Here's how the part is built. I have some questions about the finished solid (model axes, mm). A direction names the side the tool comes from. Give positions to 0.01 mm unless a question says otherwise; leave off trailing zeros. Write each loop counter-clockwise with the first axis right and the second up, starting at its lowest first coordinate (ties: lowest second). Pieces come first, ordered by that corner, then holes. Notation, with made-up numbers: (45, 22.25) -> (88, 22.25) arc R21 cw to (88, 34.25) -> close; hole circle Ø11 at (5, -2). An arc over 180 degrees is marked (long way). Use one line per item in the form item = value.
```python
from build123d import *

# Parameters (mm, degrees)
F0_W      = 11.8
F0_H      = 21.82
F3_W      = 1.2
F3_H      = 40
F4_DEPTH  = 26
F5_R      = 11.8
F6_DEPTH  = 30
F2_W      = 11.2
F2_H      = 8
F9_W      = 21
F9_H      = 12
F10_DEPTH = 20
F11_R     = 5.99999
F13_R     = 1.2
F14_R     = 3
F15_DEPTH = 12.5


# Not quite as in the source:
# - a fillet or chamfer is up to 0.001 mm smaller than in the source, because OpenCascade refuses the exact size


with BuildPart() as f1:
    # F0 (on Front) → F1 (revolve)
    with BuildSketch(Plane.XZ):
        with Locations((5.9, 10.91)):
            Rectangle(F0_W, F0_H)
    revolve(axis=Axis((0, 0, 10.91), (0, 0, 1)))


with BuildPart() as f4:
    # F3 (on Top) → F4 (new body)
    with BuildSketch(Plane.XY):
        with Locations((5.2, 0)):
            Rectangle(F3_W, F3_H)
    extrude(amount=F4_DEPTH)


with BuildPart() as f6_tool:
    # F5 (on Top) → F6 (new body)
    with BuildSketch(Plane.XY):
        Circle(F5_R)
    extrude(amount=F6_DEPTH)


with BuildPart() as f1_1:
    add(f1.part)

    # F6: intersect by f6_tool
    add(f6_tool.part, mode=Mode.INTERSECT)


with BuildPart() as f4_1:
    add(f4.part)

    # F6: intersect by f6_tool
    add(f6_tool.part, mode=Mode.INTERSECT)

    # F7: union F1
    add(f1_1.part)

    # F2 (on Front) → F8 (revolve, cut)
    with BuildSketch(Plane.XZ):
        with Locations((5.6, 4)):
            Rectangle(F2_W, F2_H)
    revolve(axis=Axis((0, 0, 4), (0, 0, 1)), mode=Mode.SUBTRACT)


with BuildPart() as f10:
    # F9 (on Top) → F10 (new body)
    with BuildSketch(Plane.XY):
        Rectangle(F9_W, F9_H)
    extrude(amount=F10_DEPTH)

    # F11 (radius 6 in the source; OpenCascade refuses exactly that, so slightly less here)
    f11_edges = [f10.edges().sort_by_distance(p)[0] for p in [
        (-10.5, -6, 10),
        (10.5, -6, 10),
        (-10.5, 6, 10),
        (10.5, 6, 10),
    ]]
    fillet(f11_edges, radius=F11_R)


with BuildPart() as f4_2:
    add(f4_1.part)

    # F12: cut F10
    add(f10.part, mode=Mode.SUBTRACT)

    # F13
    f13_edges = [f4_2.edges().sort_by_distance(p)[0] for p in [
        (4.6, 0, 21.82),
        (5.8, 0, 21.82),
    ]]
    fillet(f13_edges, radius=F13_R)

    # F14 (on Front) → F15 (cut, symmetric)
    with BuildSketch(Plane.XZ):
        with Locations((0, 12)):
            Circle(F14_R)
    extrude(amount=F15_DEPTH, both=True, mode=Mode.SUBTRACT)


solid = f4_2.part
```
Q1. If I drill on line 1 along Y through (x, z) = (0, 6); line 2 along Z through (x, y) = (2.5, -1.5); line 3 along Z through (x, y) = (2, 6.5), over which ranges is the centre line in solid material (lowest first)? Write a range as from..to.
Result set:
line_1 = -11.8..-11.2, 11.2..11.8
line_2 = 20..21.82
line_3 = 8..9.76, 14.24..21.82
Q2. I want a section at A-A, the plane x = 0. Write out the boundary of the cut face in (y, z), and give its area (3 significant figures).
Result set:
outline = (-11.8, 0) -> (-11.2, 0) -> (-11.2, 8) -> (-6, 8) -> (-6, 9) -> (-11.8, 9) -> close; (-11.8, 15) -> (-6, 15) -> (-6, 20) -> (6, 20) -> (6, 15) -> (11.8, 15) -> (11.8, 21.82) -> (-11.8, 21.82) -> close; (6, 8) -> (11.2, 8) -> (11.2, 0) -> (11.8, 0) -> (11.8, 9) -> (6, 9) -> close
area = 122 mm2
Q3. Which directions (+Z, -Z, +X, -X, +Y, -Y) give clear straight access to the entire face, cutting with the end or side of a thin tool? Please do faces 5 (the face through (-7, 9, 0)), 6 (the face through (4.6, 0, 24)), 7 (the face through (-8.789, -4.196, 14.084)).
Result set:
face_5 = -Z, +X, -X, +Y, -Y
face_6 = +Z, -X, +Y, -Y
face_7 = -Z
Q4. Will these pins go through, and if not, where does the flat tip stop? pin 1 Ø12 at (y, z) = (-8.5, 8) entering from -X; pin 2 Ø6 at (x, y) = (1, -4.5) entering from -Z; pin 3 Ø4 at (x, y) = (-6.5, 1.5) entering from -Z; pin 4 Ø5.5 at (x, z) = (0, 12) entering from +Y.
Result set:
pin_1 = -11.53
pin_2 = 8
pin_3 = 20
pin_4 = through
Q5. If we mould it in two halves opening along X, with no side actions, what happens to faces 1 (the face through (8.696, -4.289, 14.084)), 2 (the face through (-11.19, 0.49, 4.06)), 3 (the face through (5.8, 0, 24)), 4 (the face through (9, 0, 21.82))? For each: +X half, -X half, draft (parallel to the pull), parting line (faces both ways), or undercut.
Result set:
face_1 = undercut
face_2 = undercut
face_3 = +X half
face_4 = draft
Q6. I want a section at D-D, the plane y = 7.75. Write out the boundary of the cut face in (x, z).
Result set:
outline = (-8.9, 0) -> (-8.09, 0) -> (-8.09, 8) -> (8.09, 8) -> (8.09, 0) -> (8.9, 0) -> (8.9, 21.82) -> (7, 21.82) arc R1.2 cw to (5.8, 23.02) -> (5.8, 26) -> (4.6, 26) -> (4.6, 23.02) arc R1.2 cw to (3.4, 21.82) -> (-8.9, 21.82) -> close; hole circle Ø6 at (0, 12)
